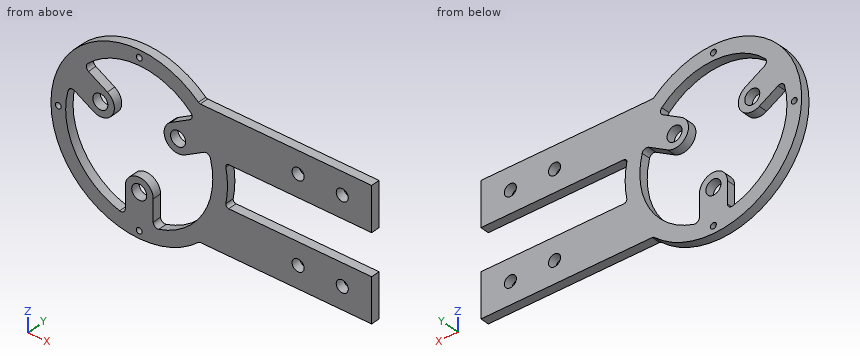
from build123d import *

# Parameters (mm, degrees)
SKETCH1_R           = 30
SKETCH1_R_2         = 25
BOSS_EXTRUDE1_DEPTH = 3
BOSS_EXTRUDE2_START = -3
SKETCH2_R           = 2.55
BOSS_EXTRUDE2_DEPTH = 3
CIRPATTERN1_COUNT   = 3
FILLET1_R           = 1.5
BOSS_EXTRUDE3_START = -3
BOSS_EXTRUDE3_DEPTH = 3
SKETCH4_R           = 2.05
CUT_EXTRUDE1_DEPTH  = 85.557672626
SKETCH5_R           = 1
CUT_EXTRUDE2_DEPTH  = 85.557672626
FILLET2_R           = 1


with BuildPart() as part:
    # Sketch1 → Boss-Extrude1 (new body)
    with BuildSketch(Plane(origin=(0, 0, 0), x_dir=(1, 0, 0), z_dir=(0, 1, 0))):
        with Locations(Location((0, 0, 0), (0, 0, 270))):
            Circle(SKETCH1_R)
        with Locations(Location((0, 0, 0), (0, 0, 270))):
            Circle(SKETCH1_R_2, mode=Mode.SUBTRACT)
    extrude(amount=BOSS_EXTRUDE1_DEPTH)

    # Sketch2 → Boss-Extrude2 (add)
    with BuildSketch(Plane(origin=(0, 3, 0), x_dir=(1, 0, 0), z_dir=(0, 1, 0)).offset(BOSS_EXTRUDE2_START)):
        with BuildLine():
            Line((-4.75, 15.25), (-4.75, 24.544602258))
            ThreePointArc((-4.75, 24.544602258), (0, 25), (4.75, 24.544602258))
            Line((4.75, 24.544602258), (4.75, 15.25))
            ThreePointArc((4.75, 15.25), (0, 10.5), (-4.75, 15.25))
        make_face()
        with Locations(Location((0, 15.25, 0), (0, 0, 270))):
            Circle(SKETCH2_R, mode=Mode.SUBTRACT)
    boss_extrude2 = extrude(amount=BOSS_EXTRUDE2_DEPTH)

    # CirPattern1: Boss-Extrude2 ×3 about axis
    cirpattern1_axis = Axis((0, 0, 0), (0, 1, 0))
    for i in range(1, CIRPATTERN1_COUNT):
        add(boss_extrude2.rotate(cirpattern1_axis, i * 360 / CIRPATTERN1_COUNT))

    # Fillet1
    fillet1_edges = [part.edges().sort_by_distance(p)[0] for p in [
        (4.75, 1.5, -24.544602258),
        (-4.75, 1.5, -24.544602258),
        (18.881249081, 1.5, 16.385921797),
        (23.631249081, 1.5, 8.158680461),
        (-23.631249081, 1.5, 8.158680461),
        (-18.881249081, 1.5, 16.385921797),
    ]]
    fillet(fillet1_edges, radius=FILLET1_R)

    # Sketch3 → Boss-Extrude3 (add)
    with BuildSketch(Plane(origin=(0, 3, 0), x_dir=(1, 0, 0), z_dir=(0, 1, 0)).offset(BOSS_EXTRUDE3_START)):
        with BuildLine():
            Line((20.396078054, 22), (79, 22))
            Line((79, 22), (79, 7))
            Line((79, 7), (29.171904292, 7))
            ThreePointArc((29.171904292, 7), (25.893941733, 15.149382216), (20.396078054, 22))
        make_face()
        with BuildLine():
            Line((29.171904292, -7), (79, -7))
            Line((79, -7), (79, -22))
            Line((79, -22), (20.396078054, -22))
            ThreePointArc((20.396078054, -22), (25.893941733, -15.149382216), (29.171904292, -7))
        make_face()
    extrude(amount=BOSS_EXTRUDE3_DEPTH)

    # Sketch4 → Cut-Extrude1 (cut, through all)
    with BuildSketch(Plane(origin=(0, 3, 0), x_dir=(1, 0, 0), z_dir=(0, 1, 0))):
        with Locations(Location((54, 14.5, 0), (0, 0, 270))):
            Circle(SKETCH4_R)
        with Locations(Location((69, 14.5, 0), (0, 0, 270))):
            Circle(SKETCH4_R)
        with Locations(Location((54, -14.5, 0), (0, 0, 270))):
            Circle(SKETCH4_R)
        with Locations(Location((69, -14.5, 0), (0, 0, 270))):
            Circle(SKETCH4_R)
    extrude(amount=-CUT_EXTRUDE1_DEPTH, mode=Mode.SUBTRACT)

    # Sketch5 → Cut-Extrude2 (cut, through all)
    with BuildSketch(Plane(origin=(0, 3, 0), x_dir=(1, 0, 0), z_dir=(0, 1, 0))):
        with Locations(Location((0, 27.5, 0), (0, 0, 270))):
            Circle(SKETCH5_R)
        with Locations(Location((-27.5, 0, 0), (0, 0, 270))):
            Circle(SKETCH5_R)
        with Locations(Location((0, -27.5, 0), (0, 0, 270))):
            Circle(SKETCH5_R)
    extrude(amount=-CUT_EXTRUDE2_DEPTH, mode=Mode.SUBTRACT)

    # Fillet2
    fillet2_edges = [part.edges().sort_by_distance(p)[0] for p in [
        (20.396078054, 1.5, 22),
        (29.171904292, 1.5, 7),
        (29.171904292, 1.5, -7),
        (20.396078054, 1.5, -22),
    ]]
    fillet(fillet2_edges, radius=FILLET2_R)


solid = part.part
The listing builds one solid part. Answer for the finished solid, in the listing's coordinates (mm). Round coordinates to 2 decimals unless told otherwise and drop trailing zeros. Order: outer loops, then holes, each group sorted by start corner. A loop starts at its lowest first (then second) coordinate and runs counter-clockwise, first axis right, second up. Notation, with made-up numbers: (-18, 75.5) - (7, 75.5) arc R22 ccw to (7, 85.5) - close; hole circle Ø11 at (-37, 26). An arc over 180 degrees is marked (long way). Write item = value, one per line. Start each with the question number.
1) Straight lines are drawn through the part: L1, parallel to Z at x = 60.5, y = 0.75; L2, parallel to X at y = 0.25, z = -23; L3, parallel to X at y = 1.95, z = 14.5. For each, find the intervals that lie inside material, in ascending order.
2) Section B-B, the plane x = 0 is taken. Write down the section's boundary in (y, z).
3) Section C-C, the plane z = 27.5 is taken. Write down the section's boundary in (x, y).
4) Given pin 1 (2.5 mm diameter, centred on x = 0, z = 27.5, fed in from +Y); pin 2 (4 mm diameter, centred on x = 13.21, z = 7.63, fed in from +Y); pin 3 (1.5 mm diameter, centred on x = 66.5, y = 1.5, fed in from -Z); pin 4 (1.5 mm diameter, centred on y = 2, z = 6, fed in from +X), each flat-ended and moving along its own axis, determine where each tip first touches the part or whether it passes through.
5) Section D-D, the plane x = -27.5 is taken. Write down the section's boundary in (y, z).
6) Section A-A, the plane x = 54 is taken. Write down the section's boundary in (y, z).
Results list:
q1.L1 = -22 to -7, 7 to 22
q1.L2 = -19.26 to -9.8, -4.79 to 4.79, 9.8 to 19.26
q1.L3 = -26.26 to -15.61, 15.61 to 51.95, 56.05 to 66.95, 71.05 to 79
q2.outline = (0, -30) - (3, -30) - (3, -28.5) - (0, -28.5) - close; (0, -26.5) - (3, -26.5) - (3, -17.8) - (0, -17.8) - close; (0, -12.7) - (3, -12.7) - (3, -10.5) - (0, -10.5) - close; (0, 25) - (3, 25) - (3, 26.5) - (0, 26.5) - close; (0, 28.5) - (3, 28.5) - (3, 30) - (0, 30) - close
q3.outline = (-11.99, 0) - (-1, 0) - (-1, 3) - (-11.99, 3) - close; (1, 0) - (11.99, 0) - (11.99, 3) - (1, 3) - close
q4.pin_1 = 3
q4.pin_2 = through
q4.pin_3 = -22
q4.pin_4 = 29.75
q5.outline = (0, -11.99) - (3, -11.99) - (3, -1) - (0, -1) - close; (0, 1) - (3, 1) - (3, 11.99) - (0, 11.99) - close
q6.outline = (0, -22) - (3, -22) - (3, -16.55) - (0, -16.55) - close; (0, -12.45) - (3, -12.45) - (3, -7) - (0, -7) - close; (0, 7) - (3, 7) - (3, 12.45) - (0, 12.45) - close; (0, 16.55) - (3, 16.55) - (3, 22) - (0, 22) - close
